Source: CAD feature listing. Evaluate the final solid. Frame: model axes, mm. Face numbers are marked on the shaded views. A direction names the side the tool comes from. Round coordinates to 2 decimals unless told otherwise and drop trailing zeros.
(1) Material intervals for probe 1 along Z at (x, y) = (0.5, -0.1); probe 2 along X at (y, z) = (-1.1, 1.85); probe 3 along Y at (x, z) = (0.75, 1), sorted ascending.
(2) First-contact query: pin 1 Ø1.5 at (y, z) = (0.5, -1) entering from -X; pin 2 Ø3 at (x, y) = (5.5, -2) entering from +Z; pin 3 Ø1.5 at (x, z) = (5, 0.5) entering from -Y. Flat tips, straight axial feed; report the tip coordinate or a pass-through.
(3) Mould query, pull axis Y, two halves, no side actions, for the marked faces 1, 2, 3 and 4. Classes: pulls with the +Y half, pulls with the -Y half, needs draft (parallel to the pull), parting line crosses it, or undercut.
(4) Set-up query: the marked faces 5 and 6. Return all of +Z, -Z, +X, -X, +Y, -Y with unobstructed straight access to the full face (end or side cutting, diameter ignored); none if empty.
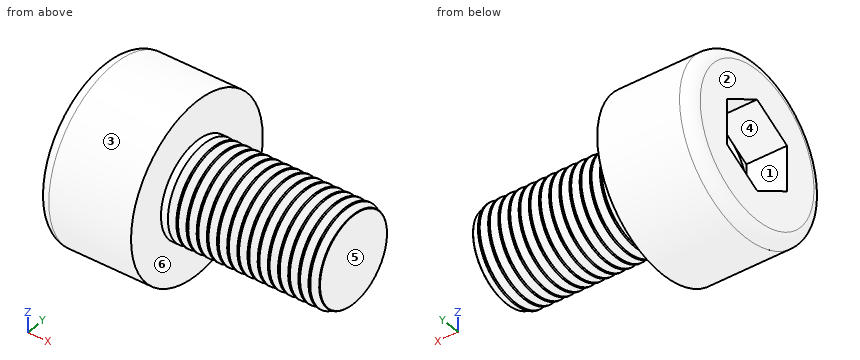
```python
from build123d import *

# Parameters (mm, degrees)
SKETCH1_R           = 2.75
BASEHEAD_DEPTH      = 3
SKETCH2_R           = 1.5
BASEBODY_DEPTH      = 5
HEXAGONSOCKET_DEPTH = 1.3
TOPFILLET_R         = 0.375
CHAMFER1_SIZE       = 0.1
LPATTERN10_COUNT    = 15
LPATTERN10_PITCH    = 0.3246


with BuildPart() as part:
    # Sketch1 → BaseHead (new body)
    with BuildSketch(Plane(origin=(0, 0, 0), x_dir=(0, 0, -1), z_dir=(1, 0, 0))):
        Circle(SKETCH1_R)
    extrude(amount=BASEHEAD_DEPTH)

    # Sketch2 → BaseBody (add)
    with BuildSketch(Plane(origin=(3, 0, 0), x_dir=(0, 0, -1), z_dir=(1, 0, 0))):
        Circle(SKETCH2_R)
    extrude(amount=BASEBODY_DEPTH)

    # Sketch3 → HexagonSocket (cut)
    with BuildSketch(Plane(origin=(0, 0, 0), x_dir=(0, 0, -1), z_dir=(1, 0, 0))):
        Polygon((1.443375673, 0), (0.721687836, 1.25), (-0.721687836, 1.25), (-1.443375673, 0), (-0.721687836, -1.25), (0.721687836, -1.25), align=None)
    extrude(amount=HEXAGONSOCKET_DEPTH, mode=Mode.SUBTRACT)

    # Sketch4 → Cut-Revolve1 (revolve, cut)
    with BuildSketch(Plane(origin=(-4.19613823, 0.75, 0), x_dir=(-1, 0, 0), z_dir=(0, 0, 1))):
        Polygon((-5.49613823, 2), (-6.217826066, 0.75), (-5.49613823, 0.75), align=None)
    revolve(axis=Axis((0.838992387, 0, 0), (-1, 0, 0)), mode=Mode.SUBTRACT)

    # TopFillet
    topfillet_edges = [part.edges().sort_by_distance(p)[0] for p in [
        (0, 0, 2.75),
    ]]
    fillet(topfillet_edges, radius=TOPFILLET_R)

    # Chamfer1
    chamfer1_edges = [part.edges().sort_by_distance(p)[0] for p in [
        (8, 0, 1.5),
    ]]
    chamfer(chamfer1_edges, length=CHAMFER1_SIZE)

    # Sketch5 → Cut-Revolve10 (revolve, cut)
    with BuildSketch(Plane.XY):
        Polygon((7.9, 1.265740128), (8.03525, 1.5), (8.03525, 1.7705), (7.76475, 1.7705), (7.76475, 1.5), align=None)
    cut_revolve10 = revolve(axis=Axis((0, 0, 0), (1, 0, 0)), mode=Mode.SUBTRACT)

    # LPattern10: Cut-Revolve10 ×15
    with Locations(*[(-i * LPATTERN10_PITCH, 0, 0) for i in range(1, LPATTERN10_COUNT)]):
        add(cut_revolve10, mode=Mode.SUBTRACT)


solid = part.part
```
Output values:
1. probe 1: z = -2.75 to -1.39, 1.39 to 2.75
1. probe 2: x = 0 to 3
1. probe 3: y = -2.56 to -0.77, 0.77 to 2.56
2. pin 1: stops at x = 0
2. pin 2: stops at z = 1.41
2. pin 3: stops at y = -1.5
3. face 1: undercut
3. face 2: needs draft
3. face 3: parting line crosses it
3. face 4: undercut
4. face 5: +Z, -Z, +X, +Y, -Y
4. face 6: +X
